from build123d import *

# Parameters (mm, degrees)
F1_DEPTH = 12.7
F2_R     = 5.905857
F3_DEPTH = 25.4


with BuildPart() as f1:
    # F0 (on Top) → F1 (new body)
    with BuildSketch(Plane.XY):
        with BuildLine():
            Line((0, 48.02762), (0, 0))
            Line((0, 0), (10.74041, 0))
            Line((10.74041, 0), (10.74041, 20.030156))
            Line((10.74041, 20.030156), (19.187918, 0))
            Line((19.187918, 0), (30.046732, 0))
            Line((30.046732, 0), (18.06753, 24.186372))
            ThreePointArc((18.06753, 24.186372), (23.922272, 47.389901), (0, 48.02762))
        make_face()
    extrude(amount=F1_DEPTH)

    # F2 (on face) → F3 (cut)
    with BuildSketch(Plane.XY.offset(12.7)):
        with Locations((12.875857, 40.980149)):
            Circle(F2_R)
    extrude(amount=-F3_DEPTH, mode=Mode.SUBTRACT)


solid = f1.part
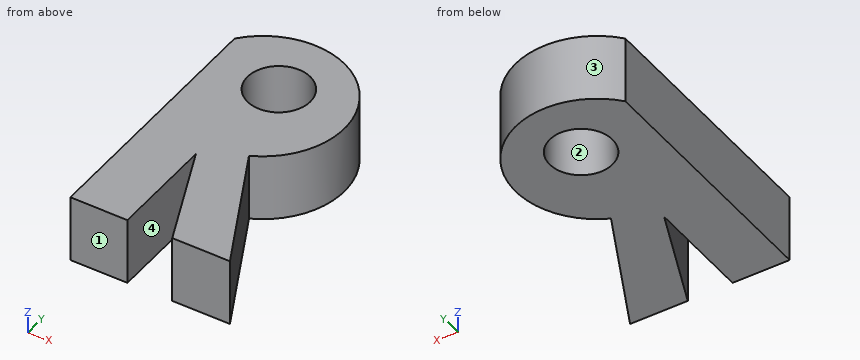
Can you work these out from the model? Positions are in its coordinate system, mm. Face numbers are marked on the shaded views. Round coordinates to 2 decimals unless told otherwise and drop trailing zeros. Order: outer loops, then holes, each group sorted by start corner. A loop starts at its lowest first (then second) coordinate and runs counter-clockwise, first axis right, second up. Notation, with made-up numbers: (-35.75, 24) -> (20.25, 24) arc R10 ccw to (20.25, 35) -> close; hole circle Ø7 at (70.25, 30). An arc over 180 degrees is marked (long way). Write each question's results on one line, items separated by ' | '. Start each with the question number.
Item 1: If we section it at B-B, the plane x = 24.5: Write out the boundary of the cut face in (y, z), then the cut area to 3 significant figures.
Item 2: Will these pins go through, and if not, where does the flat tip stop? pin 1 (6 mm diameter, centred on x = 25, y = 11.5, fed in from -Z); pin 2 (5 mm diameter, centred on x = 23.5, z = 1.5, fed in from +Y).
Item 3: If we section it at C-C, the plane z = 7: Write out the boundary of the cut face in (x, y).
Item 4: Please list where these lines run through material, in increasing order: L1, parallel to X at y = 36, z = 8.75; L2, parallel to X at y = 43, z = 1; L3, parallel to Y at x = 24, z = 8.25.
Item 5: Thinking about a two-plate mould opening in Y: for the marked faces 1, 2, 3 and 4, which applies, +Y half, -Y half, draft (parallel to the pull), parting line (faces both ways), or undercut?
Item 6: If we section it at A-A, the plane y = 12: Write out the boundary of the cut face in (x, z).
Item 7: If we section it at D-D, the plane x = 4: Write out the boundary of the cut face in (y, z), then the cut area to 3 significant figures.
Results:
1) outline: (0, 0) -> (11.2, 0) -> (11.2, 12.7) -> (0, 12.7) -> close; (29.69, 0) -> (46.57, 0) -> (46.57, 12.7) -> (29.69, 12.7) -> close | area: 357 mm2
2) pin 1: stops at z = 0 | pin 2: stops at y = 50.32
3) outline: (0, 0) -> (10.74, 0) -> (10.74, 20.03) -> (19.19, 0) -> (30.05, 0) -> (18.07, 24.19) arc R15.33 ccw (long way) to (0, 48.03) -> close; hole circle Ø11.81 at (12.88, 40.98)
4) L1: x = 0 to 9.7, 16.05 to 26.88 | L2: x = 0 to 7.33, 18.43 to 26.24 | L3: y = 0 to 12.21, 28.98 to 47.29
5) face 1: -Y half | face 2: undercut | face 3: undercut | face 4: draft
6) outline: (0, 0) -> (10.74, 0) -> (10.74, 12.7) -> (0, 12.7) -> close; (14.13, 0) -> (24.1, 0) -> (24.1, 12.7) -> (14.13, 12.7) -> close
7) outline: (0, 0) -> (51.38, 0) -> (51.38, 12.7) -> (0, 12.7) -> close | area: 653 mm2
